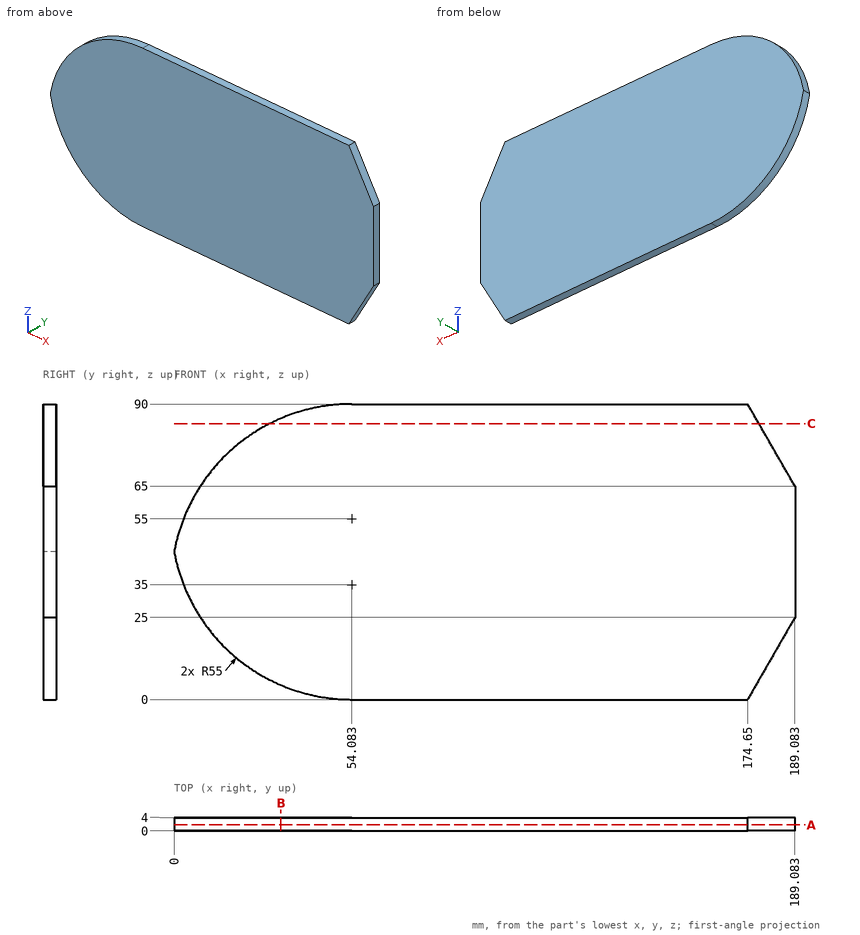
Drawing for the job (mm, zero at the part's lowest x, y, z). Coordinates: 2 decimals unless noted, no trailing zeros. Write each loop counter-clockwise with the first axis right and the second up, starting at its lowest first coordinate (ties: lowest second). Pieces come first, ordered by that corner, then holes. Notation, with made-up numbers: (46, -25.75) - (75, -25.75) arc R31 ccw to (75, 1.25) - close; hole circle Ø6 at (25, -1). An arc over 180 degrees is marked (long way). Write each question's results on one line, items separated by ' | '. Start each with the question number.
1) Probe line 1 along X through (y, z) = (0.75, 64.5) (1 decimal); line 2 along Z through (x, y) = (18, 1.6); line 3 along X through (y, z) = (1.15, 81.5) (1 decimal). List the from-to ranges inside material, lowest first. Write a range as from..to.
2) Cut at C-C (z = 84). Write the cut outline in (x, y), then the cut area to 3 significant figures.
3) Cut at A-A (y = 1.75). Write the cut outline in (x, z), then the cut area to 3 significant figures.
4) Cut at B-B (x = 32.5). Write the cut outline in (y, z).
Returned:
1) line 1: 7.7..189.1 | line 2: 13.49..76.51 | line 3: 24.7..179.6
2) outline: (29.1, 0) - (178.11, 0) - (178.11, 4) - (29.1, 4) - close | area: 596 mm^2
3) outline: (0, 45) arc R55 ccw to (54.08, 0) - (174.65, 0) - (189.08, 25) - (189.08, 65) - (174.65, 90) - (54.08, 90) arc R55 ccw to start | area: 15,400 mm^2
4) outline: (0, 4.41) - (4, 4.41) - (4, 85.59) - (0, 85.59) - close
